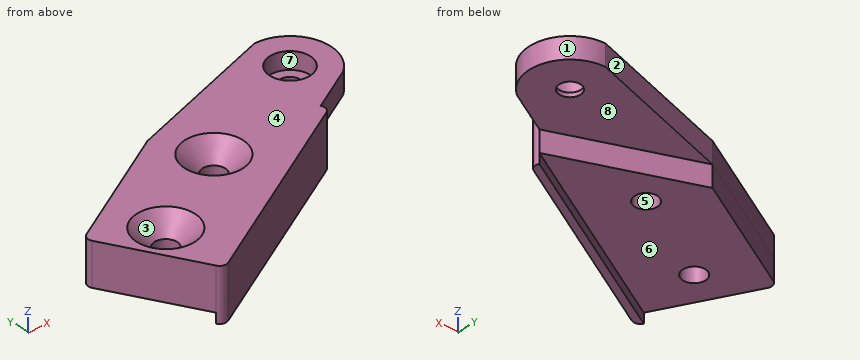
```python
from build123d import *

# Parameters (mm, degrees)
SKETCH4_R           = 1.6
BOSS_EXTRUDE1_DEPTH = 3
BOSS_EXTRUDE2_DEPTH = 1.4
SKETCH6_R           = 1.6
BOSS_EXTRUDE3_DEPTH = 3
SKETCH7_R           = 2.85
CUT_EXTRUDE1_DEPTH  = 2.4
CUT_EXTRUDE2_DEPTH  = 4.6
SKETCH10_R          = 1.5
CUT_EXTRUDE3_DEPTH  = 10
CHAMFER1_SIZE       = 2.5
FILLET1_R           = 1


with BuildPart() as part:
    # Sketch4 → Boss-Extrude1 (new body)
    with BuildSketch(Plane.XY):
        Polygon((263.556481558, 184.695050819), (264.03563075, 183.817317345), (235.433373737, 168.203524869), (234.954224546, 169.081258344), (227.766986674, 182.247260462), (245.321656165, 191.830244291), align=None)
        with Locations((235.749272983, 178.06000536)):
            Circle(SKETCH4_R, mode=Mode.SUBTRACT)
        with Locations((248.915275101, 185.247243232)):
            Circle(SKETCH4_R, mode=Mode.SUBTRACT)
    extrude(amount=BOSS_EXTRUDE1_DEPTH)

    # Sketch5 → Boss-Extrude2 (add)
    with BuildSketch(Plane(origin=(0, 0, 0), x_dir=(-1, 0, 0), z_dir=(0, 0, -1))):
        Polygon((-263.556481558, 184.695050819), (-264.03563075, 183.817317345), (-235.433373737, 168.203524869), (-234.954224546, 169.081258344), align=None)
    extrude(amount=BOSS_EXTRUDE2_DEPTH)

    # Sketch6 → Boss-Extrude3 (add)
    with BuildSketch(Plane.XY.offset(3)):
        with BuildLine():
            Line((227.766986674, 182.247260462), (257.291019991, 198.364244833))
            Line((257.291019991, 198.364244833), (266.21359493, 198.317204861))
            ThreePointArc((266.21359493, 198.317204861), (271.61517707, 194.425420779), (269.70061588, 188.049095159))
            Line((269.70061588, 188.049095159), (263.556481558, 184.695050819))
            Line((263.556481558, 184.695050819), (264.03563075, 183.817317345))
            Line((264.03563075, 183.817317345), (235.433373737, 168.203524869))
            Line((235.433373737, 168.203524869), (234.954224546, 169.081258344))
            Line((234.954224546, 169.081258344), (227.766986674, 182.247260462))
        make_face()
        with Locations((248.915275101, 185.247243232)):
            Circle(SKETCH6_R, mode=Mode.SUBTRACT)
        with Locations((235.749272983, 178.06000536)):
            Circle(SKETCH6_R, mode=Mode.SUBTRACT)
    extrude(amount=BOSS_EXTRUDE3_DEPTH)

    # Sketch7 → Cut-Extrude1 (cut)
    with BuildSketch(Plane.XY.offset(6)):
        with Locations((266.183352442, 192.580788532)):
            Circle(SKETCH7_R)
    extrude(amount=-CUT_EXTRUDE1_DEPTH, mode=Mode.SUBTRACT)

    # Sketch9 → Cut-Extrude2 (cut)
    with BuildSketch(Plane(origin=(0, 0, 3), x_dir=(-1, 0, 0), z_dir=(0, 0, -1))):
        Polygon((-245.321656165, 191.830244291), (-266.21359493, 198.317204861), (-257.291019991, 198.364244833), align=None)
    extrude(amount=-CUT_EXTRUDE2_DEPTH, mode=Mode.SUBTRACT)

    # Sketch10 → Cut-Extrude3 (cut)
    with BuildSketch(Plane.XY.offset(3.6)):
        with Locations((266.183352442, 192.580788532)):
            Circle(SKETCH10_R)
    extrude(amount=-CUT_EXTRUDE3_DEPTH, mode=Mode.SUBTRACT)

    # Chamfer1
    chamfer1_edges = [part.edges().sort_by_distance(p)[0] for p in [
        (247.315275101, 185.247243232, 6),
        (234.149272983, 178.06000536, 6),
    ]]
    chamfer(chamfer1_edges, length=CHAMFER1_SIZE)

    # Fillet1
    fillet1_edges = [part.edges().sort_by_distance(p)[0] for p in [
        (264.03563075, 183.817317345, 2.3),
        (227.766986674, 182.247260462, 3),
        (235.433373737, 168.203524869, 2.3),
    ]]
    fillet(fillet1_edges, radius=FILLET1_R - 0.0001)  # a hair under: the kernel refuses the full size


solid = part.part
```
Geometry check sheet. Reference: the model listing, model coordinates, mm. Face numbers are marked on the shaded views. A direction names the side the tool comes from. Give positions to 0.01 mm unless a question says otherwise; leave off trailing zeros. Loops run counter-clockwise (first coordinate to the right, second up) from the corner with the lowest first, then second, coordinate; pieces in that order, holes last. Notation, with made-up numbers: M 11.5,34.5 L 18.5,34.5 A26 ccw 18.5,56.5 Z; hole C 15.25,70 d6. An arc over 180 degrees is marked long. Write item = value, one per line. Start each with the question number.
1. Section check B-B, the plane x = 259. Enter the section's corners in (y, z), plus the area to 3 significant figures.
2. Draft check along X on the marked faces 1, 2 and 3. Enter one of: +X half, -X half, draft (parallel to the pull), parting line (faces both ways), or undercut.
3. Go/stop test with flat-tipped pins: P1, Ø1.9, axis at x = 248.92, y = 185.25, coming from the +Z side; P2, Ø7, axis at x = 253.5, y = 191, coming from the -Z side; P3, Ø3, axis at x = 246, z = 4, coming from the +Y side; P4, Ø3, axis at x = 264.5, y = 192.5, coming from the -Z side. Record where each tip stops, or that it passes through.
4. Tool access check on the marked faces 4, 5, 6, 7 and 8. Record the directions out of +Z, -Z, +X, -X, +Y, -Y that give a thin tool (end or side, any length) a straight path to the whole face; none if there is none.
5. Section check A-A, the plane z = 4.25. Give the number of separate pieces and of enclosed holes in the cut face, plus the area to 3 significant figures.
6. Thickness scan on probe 1 along Z at (x, y) = (260.5, 188); probe 2 along X at (y, z) = (184, 1.25); probe 3 along Z at (x, y) = (243, 181.5). Record the ranges inside material, lowest first.
Values follow:
q1.outline = M 181.07,-1.4 L 182.21,-1.4 L 182.21,0 L 186.48,0 L 186.48,3 L 196.08,3 L 196.08,6 L 181.07,6 Z
q1.area = 62.9 mm^2
q2.face_1 = +X half
q2.face_2 = -X half
q2.face_3 = undercut
q3.P1 = through
q3.P2 = 0
q3.P3 = 192.51
q3.P4 = 3
q4.face_4 = +Z, +X, -X, +Y, -Y
q4.face_5 = +Z, -Z
q4.face_6 = -Z, -X, +Y
q4.face_7 = +Z
q4.face_8 = -Z, +X, +Y
q5.separate_pieces = 1
q5.enclosed_holes = 3
q5.area = 568 mm^2
q6.probe_1 = 3 to 6
q6.probe_2 = 230.98 to 247.91, 249.92 to 263.66
q6.probe_3 = 0 to 6
